from build123d import *

# Parameters (mm, degrees)
SKETCH1_W             = 139.7
SKETCH1_H             = 57.15
BOSS_EXTRUDE1_DEPTH   = 25.4
FILLET1_R             = 6.35
SKETCH5_W             = 133.35
SKETCH5_H             = 50.8
CUT_EXTRUDE1_DEPTH    = 23.8125
FILLET5_R             = 12.7
F_4_CLEARANCE_HOLE1_D = 2.9464
FILLET6_R             = 1.5875
CUT_EXTRUDE2_REACH    = 146.837
SKETCH6_W             = 20.32
SKETCH6_H             = 7.62
CUT_EXTRUDE3_REACH    = 95.757
SKETCH7_W             = 20.32
SKETCH7_H             = 7.62
CUT_EXTRUDE4_REACH    = 95.757
SKETCH8_W             = 12.7
SKETCH8_H             = 10.16
FILLET7_R             = 3.175
CUT_EXTRUDE5_REACH    = 95.757
SKETCH9_W             = 12.7
SKETCH9_H             = 10.16
FILLET9_R             = 3.175


with BuildPart() as part:
    # Sketch1 → Boss-Extrude1 (new body)
    with BuildSketch(Plane(origin=(0, 0, 0), x_dir=(1, 0, 0), z_dir=(0, 1, 0))):
        Rectangle(SKETCH1_W, SKETCH1_H)
    extrude(amount=BOSS_EXTRUDE1_DEPTH)

    # Fillet1
    fillet1_edges = [part.edges().sort_by_distance(p)[0] for p in [
        (69.85, 12.7, 28.575),
        (-69.85, 12.7, 28.575),
        (-69.85, 12.7, -28.575),
        (69.85, 12.7, -28.575),
    ]]
    fillet(fillet1_edges, radius=FILLET1_R)

    # Sketch5 → Cut-Extrude1 (cut)
    with BuildSketch(Plane.XZ):
        Rectangle(SKETCH5_W, SKETCH5_H)
    extrude(amount=-CUT_EXTRUDE1_DEPTH, mode=Mode.SUBTRACT)

    # Fillet5
    fillet5_edges = [part.edges().sort_by_distance(p)[0] for p in [
        (-66.675, 11.90625, 25.4),
        (66.675, 11.90625, 25.4),
        (66.675, 11.90625, -25.4),
        (-66.675, 11.90625, -25.4),
    ]]
    fillet(fillet5_edges, radius=FILLET5_R)

    # #4 Clearance Hole1 (through all)
    with Locations(Plane(origin=(0, 25.4, 0), x_dir=(-1, 0, 0), z_dir=(0, 1, 0))):
        with Locations((64.77, -22.86), (64.77, 22.86), (-64.77, -22.86), (-64.77, 22.86)):
            Hole(F_4_CLEARANCE_HOLE1_D / 2)

    # Fillet6
    fillet6_edges = [part.edges().sort_by_distance(p)[0] for p in [
        (-69.85, 25.4, 0),
        (0, 25.4, -28.575),
        (69.85, 25.4, 0),
        (0, 25.4, 28.575),
        (-67.990128061, 25.4, 26.715128061),
        (67.990128061, 25.4, 26.715128061),
        (67.990128061, 25.4, -26.715128061),
        (-67.990128061, 25.4, -26.715128061),
    ]]
    fillet(fillet6_edges, radius=FILLET6_R)

    # Sketch6 → Cut-Extrude2 (cut, up to next)
    with BuildSketch(Plane(origin=(69.85, 0, 0), x_dir=(0, 0, -1), z_dir=(1, 0, 0)), mode=Mode.PRIVATE) as cut_extrude2_sk1:
        with Locations((0, 3.81)):
            Rectangle(SKETCH6_W, SKETCH6_H)
    cut_extrude2_tool1 = extrude(cut_extrude2_sk1.sketch, amount=-CUT_EXTRUDE2_REACH, mode=Mode.PRIVATE) & part.part
    add(cut_extrude2_tool1.solids().sort_by_distance((69.85, 3.81, 0))[0], mode=Mode.SUBTRACT)

    # Sketch7 → Cut-Extrude3 (cut, up to next)
    with BuildSketch(Plane.XY.offset(28.575), mode=Mode.PRIVATE) as cut_extrude3_sk1:
        with Locations((-38.1, 3.81)):
            Rectangle(SKETCH7_W, SKETCH7_H)
    cut_extrude3_tool1 = extrude(cut_extrude3_sk1.sketch, amount=-CUT_EXTRUDE3_REACH, mode=Mode.PRIVATE) & part.part
    add(cut_extrude3_tool1.solids().sort_by_distance((-38.1, 3.81, 28.575))[0], mode=Mode.SUBTRACT)

    # Sketch8 → Cut-Extrude4 (cut, up to next)
    with BuildSketch(Plane(origin=(0, 0, -28.575), x_dir=(-1, 0, 0), z_dir=(0, 0, -1)), mode=Mode.PRIVATE) as cut_extrude4_sk1:
        with Locations((-49.53, 5.08)):
            Rectangle(SKETCH8_W, SKETCH8_H)
    cut_extrude4_tool1 = extrude(cut_extrude4_sk1.sketch, amount=-CUT_EXTRUDE4_REACH, mode=Mode.PRIVATE) & part.part
    add(cut_extrude4_tool1.solids().sort_by_distance((49.53, 5.08, -28.575))[0], mode=Mode.SUBTRACT)

    # Fillet7
    fillet7_edges = [part.edges().sort_by_distance(p)[0] for p in [
        (68.2625, 7.62, -10.16),
        (68.2625, 7.62, 10.16),
        (-27.94, 7.62, 26.9875),
        (-48.26, 7.62, 26.9875),
        (43.18, 10.16, -26.9875),
        (55.88, 10.16, -26.915656079),
    ]]
    fillet(fillet7_edges, radius=FILLET7_R)

    # Sketch9 → Cut-Extrude5 (cut, up to next)
    with BuildSketch(Plane.XY.offset(28.575), mode=Mode.PRIVATE) as cut_extrude5_sk1:
        with Locations((0, 5.08)):
            Rectangle(SKETCH9_W, SKETCH9_H)
    cut_extrude5_tool1 = extrude(cut_extrude5_sk1.sketch, amount=-CUT_EXTRUDE5_REACH, mode=Mode.PRIVATE) & part.part
    cut_extrude5 = cut_extrude5_tool1.solids().sort_by_distance((0, 5.08, 28.575))[0]
    add(cut_extrude5, mode=Mode.SUBTRACT)

    # Mirror1: Cut-Extrude5 across plane
    add(cut_extrude5.mirror(Plane.XY), mode=Mode.SUBTRACT)

    # Fillet9
    fillet9_edges = [part.edges().sort_by_distance(p)[0] for p in [
        (6.35, 10.16, 26.9875),
        (-6.35, 10.16, 26.9875),
        (6.35, 10.16, -26.9875),
        (-6.35, 10.16, -26.9875),
    ]]
    fillet(fillet9_edges, radius=FILLET9_R)


solid = part.part
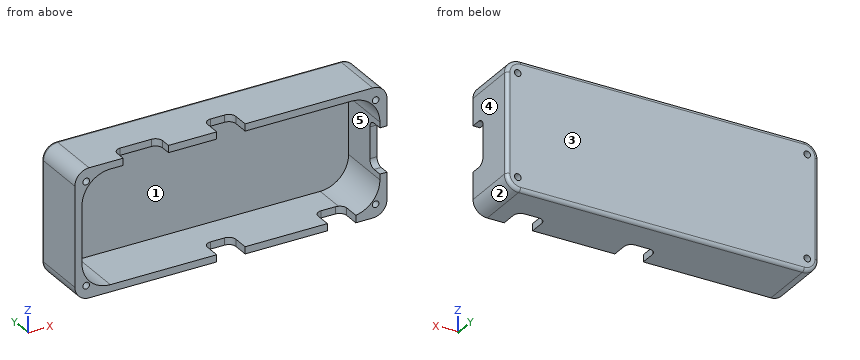
Here's how the part is built. I have some questions about the finished solid (model axes, mm). Face numbers are marked on the shaded views. A direction names the side the tool comes from. Round coordinates to 2 decimals unless told otherwise and drop trailing zeros. Loops run counter-clockwise (first coordinate to the right, second up) from the corner with the lowest first, then second, coordinate; pieces in that order, holes last. Notation, with made-up numbers: M 59.25,28.25 L 68.25,28.25 A14 ccw 68.25,49.25 Z; hole C 26,69.5 d7. An arc over 180 degrees is marked long. Write each question's results on one line, items separated by ' | '. Start each with the question number.
(1) I want a section at A-A (x = 41.5). Please give me the cut outline in (y, z) (1 decimal), then the cut area to 3 significant figures.
(2) Thinking about a two-plate mould opening in Z: for the marked faces 1, 2 and 3, which applies, pulls with the +Z half, pulls with the -Z half, needs draft (parallel to the pull), parting line crosses it, or undercut?
(3) On a 3-axis mill with a long thin cutter (end or side, diameter ignored), from which of +Z, -Z, +X, -X, +Y, -Y can I reach the whole of each face in a straight line? I mean the marked faces 4 and 5. Say none if no direction works.
(4) If I drill on probe 1 along X at (y, z) = (4, 11.5) (3 decimals); probe 2 along Z at (x, y) = (-19.5, 10.5) (3 decimals); probe 3 along Z at (x, y) = (64.77, 7.25), over which ranges is the centre line in solid material (lowest first)? Write a range as from..to.
(5) Will these pins go through, and if not, where does the flat tip stop? P1, Ø2.5, axis at x = -40, z = 27.5, coming from the -Y side; P2, Ø4, axis at x = -49, z = 2, coming from the -Y side; P3, Ø3.5, axis at y = 2, z = 27, coming from the -X side.
(6) I want a section at C-C (x = -64.77). State how many separate pieces and enclosed holes the cut face has, then the cut area to 3 significant figures.
Solved:
1) outline: M 0,-28.6 L 23.8,-28.6 A1.6 ccw 25.4,-27 L 25.4,27 A1.6 ccw 23.8,28.6 L 0,28.6 L 0,25.4 L 23.8,25.4 L 23.8,-25.4 L 0,-25.4 Z | area: 241 mm²
2) face 1: undercut | face 2: pulls with the -Z half | face 3: needs draft
3) face 4: +Z, -Z, +X, +Y, -Y | face 5: -Y
4) probe 1: x = -69.85..-66.675, 66.675..69.85 | probe 2: z = -28.575..-25.4, 25.4..28.575 | probe 3: z = -28.45..-24.33, -21.39..-19.39, 19.39..21.39, 24.33..28.45
5) P1: stops at y = 7.62 | P2: stops at y = 23.81 | P3: stops at x = -69.08
6) separate pieces: 3 | enclosed holes: 0 | area: 371 mm²
